Autodesk Fusion 360 part; units mm, degrees
sketch "Skizze1" plane through (0, 0, 0) normal (0, 0, 1) x (1, 0, 0)
  line L0 (8, 0) -> (8, 15)
  line L1 (8, 15) -> (0, 15)
  line L2 (0, 15) -> (0, -10)
  line L3 (8, 0) -> (10, 0)
  line L4 (10, 0) -> (10, 17)
  line L5 (10, 17) -> (-2, 17)
  line L6 (-2, 17) -> (-2, -10)
  line L7 (-2, -10) -> (0, -10)
  circle A0 centre (-4.9997, -10.052) radius 5
  circle A1 centre (-4.9999, -9.9716) radius 3
  line L8 (-3.9109, -5.172) -> (-4.9999, -9.9716)
  dimension "d2" = 8
  dimension "d3" = 15
  dimension "d4" = 25
  dimension "d5" = 2
  dimension "d6" = 2
  dimension "d7" = 2
  dimension "d8" = 10
  dimension "d9" = 6
extrude "Extrusion1" add sketch "Skizze1" along normal blind 10 contours L0 L1 L2 L3 L4 L5 L6 A0 | L7 A0 A1 L8 | L6 L7 A0 A1
equation "d6 = d5"
equation "d7 = d5"
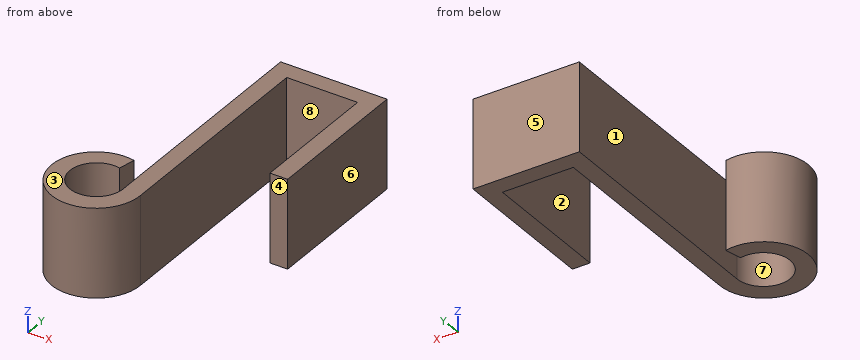
Input: part model. Units: mm. Frame: model coordinates. Face numbers are marked on the shaded views. A direction names the side the tool comes from. Give positions to 0.01 mm unless a question says otherwise; leave off trailing zeros. Order: outer loops, then holes, each group sorted by start corner. A loop starts at its lowest first (then second) coordinate and runs counter-clockwise, first axis right, second up.
1. Material intervals for L1, parallel to X at y = -10, z = 2.25; L2, parallel to X at y = 8, z = 9.5; L3, parallel to Y at x = -5, z = 7, sorted ascending.
Derived:
L1: x = -10 to -8, -2 to 0
L2: x = -2 to 0, 8 to 10
L3: y = -15.05 to -12.97, -6.97 to -5.05
2. Mould query, pull axis X, two halves, no side actions, for the marked faces 5, 6, 7 and 8. Classes: released by +X, released by -X, zero draft, split by the parting line, or undercut.
Derived:
face 5: zero draft
face 6: released by +X
face 7: undercut
face 8: undercut
3. Reachability of the marked faces 1, 2, 3 and 4 from +Z, -Z, +X, -X, +Y, -Y: full face, straight path, thin tool, end or side. Return the list, or none.
Derived:
face 1: +Z, -Z, +Y
face 2: +Z, -Z, -Y
face 3: +Z, +X, -X, +Y, -Y
face 4: +Z, -Z, +X, -Y
4. Section B-B on x = -5.75. Return the cut outline in (y, z).
Derived:
outline: (-15, 0) - (-12.88, 0) - (-12.88, 10) - (-15, 10) - close; (-7.07, 0) - (-5.11, 0) - (-5.11, 10) - (-7.07, 10) - close
5. Section D-D on x = 4. Return the cut outline in (y, z).
Derived:
outline: (15, 0) - (17, 0) - (17, 10) - (15, 10) - close
6. Section C-C on z = 2. Return the cut outline in (x, y).
Derived:
outline: (-4.34, -7.05) - (-3.91, -5.17) arc R5 ccw (long way) to (0, -10) - (0, 15) - (8, 15) - (8, 0) - (10, 0) - (10, 17) - (-2, 17) - (-2, -10) arc R3 cw (long way) to start
7. Pin query (flat end, axial travel): pin 1 (3 mm diameter, centred on x = -7, z = 5, fed in from +Y); pin 2 (5 mm diameter, centred on y = 9, z = 6.5, fed in from -X); pin 3 (1.6 mm diameter, centred on x = 9, z = 5.5, fed in from -Y); pin 4 (4 mm diameter, centred on x = -1.5, y = 2, fed in from -Z). Return the tip coordinate at first contact, or that it passes through.
Derived:
pin 1: stops at y = -5.08
pin 2: stops at x = -2
pin 3: stops at y = 0
pin 4: stops at z = 0
8. Section A-A on y = 5.5. Return the cut outline in (x, z).
Derived:
outline: (-2, 0) - (0, 0) - (0, 10) - (-2, 10) - close; (8, 0) - (10, 0) - (10, 10) - (8, 10) - close
